The listing builds one solid part. Answer for the finished solid, in the listing's coordinates (mm). A direction names the side the tool comes from. Give positions to 0.01 mm unless a question says otherwise; leave off trailing zeros. Order: outer loops, then holes, each group sorted by start corner. A loop starts at its lowest first (then second) coordinate and runs counter-clockwise, first axis right, second up. Notation, with made-up numbers: (-33.75, 42.5) - (6.25, 42.5) arc R36 cw to (6.25, 77.5) - close; hole circle Ø5 at (6.25, 65.25). An arc over 180 degrees is marked (long way). Write each question's results on one line, items separated by ' | '. Start each with the question number.
1. Determine the mould class of faces 3 (the face through (38, 0, 31)), 4 (the face through (76.2, 2, 14)), 5 (the face through (25.48, 1.61, 50.55)), 6 (the face through (22, 1.6, 21.8)) for opening direction X: released by +X, released by -X, zero draft, split by the parting line, or undercut.
2. Section D-D (y = 1.7) is taken. State how many separate pieces and enclosed holes the cut face has, and give its area (3 significant figures).
3. Flat-ended cylindrical pins translate along their axes: pin 1 (1.5 mm diameter, centred on y = 2.5, z = 26, fed in from +X); pin 2 (3.5 mm diameter, centred on x = 38.1, z = 38.1, fed in from -Y); pin 3 (1 mm diameter, centred on x = 35, y = 1, fed in from -Z); pin 4 (1 mm diameter, centred on y = 1, z = 35, fed in from -X). Find the tip coordinate at first contact, or state that the pin passes through.
4. Section C-C (x = 38.1) is taken. Give the vertices of the cut face in (y, z) (3 decimals).
5. Find the intervals of material crossed by L1, parallel to X at y = 2.1, z = 17.5; L2, parallel to X at y = 2.05, z = 38.1; L3, parallel to Z at x = 46.5, y = 0.75, in increasing order.
6. Section B-B (z = 38.1) is taken. Give the vertices of the cut face in (x, y) (3 decimals).
7. Which of the six approach directions +Z, -Z, +X, -X, +Y, -Y give full straight-line access (tool end or side, diameter ignored) to faces 1 (the face through (63.3, 1.6, 38.3)), 2 (the face through (22.098, 2, 12))?
8. Section A-A (x = 12.7) is taken. Give the vertices of the cut face in (y, z) (3 decimals), and give its area (3 significant figures).
Autodesk Fusion 360 part; units mm, degrees
sketch "Sketch1" plane through (0, 0, 0) normal (0, 1, 0) x (1, 0, 0)
  line L0 (0, 0) -> (0, -25.4)
  line L1 (76.2, -25.4) -> (76.2, 0)
  line L2 (76.2, 0) -> (54.102, 0)
  line L3 (54.102, 0) -> (54.102, -25.4)
  line L4 (54.102, -25.4) -> (22.098, -25.4)
  line L5 (22.098, -25.4) -> (22.098, 0)
  line L6 (22.098, 0) -> (0, 0)
  line L7 (38.1, -25.4) -> (38.1, -50.8) construction
  circle A0 centre (23.7818, -23.7162) radius 2.3813
  line L8 (23.7818, -23.7162) -> (23.7818, -25.4) construction
  line L9 (23.7818, -23.7162) -> (22.098, -23.7162) construction
  circle A1 centre (12.7, -12.7) radius 2.7781
  line L10 (0, -25.4) -> (25.4, -50.8)
  line L11 (25.4, -50.8) -> (50.8, -50.8)
  line L12 (50.8, -50.8) -> (76.2, -25.4)
  circle A2 centre (12.7, -25.4) radius 2.7781
  circle A3 centre (25.4, -38.1) radius 2.7781
  circle A4 centre (38.1, -38.1) radius 2.7781
  circle A5 centre (50.8, -38.1) radius 2.7781
  circle A6 centre (63.5, -12.7) radius 2.7781
  circle A7 centre (63.5, -25.4) radius 2.7781
  circle A8 centre (52.4182, -23.7162) radius 2.3813
  dimension "d1" = 76.2
  dimension "d3" = 32.004
  dimension "d4" = 25.4
  dimension "d6" = 25.4
  dimension "d8" = 4.7625
  dimension "d9" = 5.5563
  dimension "d10" = 12.7
  dimension "d26" = 25.4
  dimension "d43" = 25.4
  dimension "d44" = 12.7
  dimension "d47" = -25.4
  dimension "d48" = -50.8
extrude "Extrude1" add sketch "Sketch1" along normal blind 3.175 contours L0 L1 L2 L3 L4 L5 L6 A0 L10 L11 L12 A8
fillet "Fillet1" radius 3.175 8 edges at (0, 1.5875, 0) (22.098, 1.5875, 0) (54.102, 1.5875, 0) (76.2, 1.5875, 0) (0, 1.5875, 25.4) (25.4, 1.5875, 50.8) (50.8, 1.5875, 50.8) (76.2, 1.5875, 25.4)
fillet "Fillet1" radius 3.175 4 edges at (25.4656, 1.5875, 25.4) (22.098, 1.5875, 22.0324) (50.7344, 1.5875, 25.4) (54.102, 1.5875, 22.0324)
sketch "DXF" plane through (0, 0, 0) normal (0, -1, 0) x (1, 0, 0)
  circle A0 centre (38.1, 38.1) radius 2.7781
  circle A1 centre (12.7, 12.7) radius 2.7781
  circle A2 centre (25.4, 38.1) radius 2.7781
  circle A3 centre (12.7, 25.4) radius 2.7781
  circle A4 centre (63.5, 12.7) radius 2.7781
  circle A5 centre (63.5, 25.4) radius 2.7781
  circle A6 centre (50.8, 38.1) radius 2.7781
  arc A7 (54.5005, 22.5611) -> (54.102, 21.021) centre (57.277, 21.021) ccw
  line L0 (54.102, 21.021) -> (54.102, 3.175)
  arc A8 (54.102, 3.175) -> (57.277, 0) centre (57.277, 3.175) ccw
  line L1 (57.277, 0) -> (73.025, 0)
  arc A9 (73.025, 0) -> (76.2, 3.175) centre (73.025, 3.175) ccw
  line L2 (76.2, 3.175) -> (76.2, 24.0849)
  arc A10 (76.2, 24.0849) -> (75.2701, 26.3299) centre (73.025, 24.0849) ccw
  line L3 (75.2701, 26.3299) -> (51.7299, 49.8701)
  arc A11 (51.7299, 49.8701) -> (49.4849, 50.8) centre (49.4849, 47.625) ccw
  line L4 (49.4849, 50.8) -> (26.7151, 50.8)
  arc A12 (26.7151, 50.8) -> (24.4701, 49.8701) centre (26.7151, 47.625) ccw
  line L5 (24.4701, 49.8701) -> (0.9299, 26.3299)
  arc A13 (0.9299, 26.3299) -> (0, 24.0849) centre (3.175, 24.0849) ccw
  line L6 (0, 24.0849) -> (0, 3.175)
  arc A14 (0, 3.175) -> (3.175, 0) centre (3.175, 3.175) ccw
  line L7 (3.175, 0) -> (18.923, 0)
  arc A15 (18.923, 0) -> (22.098, 3.175) centre (18.923, 3.175) ccw
  line L8 (22.098, 3.175) -> (22.098, 21.021)
  arc A16 (22.098, 21.021) -> (21.6995, 22.5611) centre (18.923, 21.021) ccw
  arc A17 (24.9369, 25.7985) -> (21.6995, 22.5611) centre (23.7818, 23.7162) ccw
  arc A18 (24.9369, 25.7985) -> (26.477, 25.4) centre (26.477, 28.575) ccw
  line L9 (26.477, 25.4) -> (49.723, 25.4)
  arc A19 (49.723, 25.4) -> (51.2631, 25.7985) centre (49.723, 28.575) ccw
  arc A20 (54.5005, 22.5611) -> (51.2631, 25.7985) centre (52.4182, 23.7162) ccw
equation "TOLERANCE = 0.01 in"
equation "d3 = 1 in + 2 * PLATE_THICKNESS + TOLERANCE"
equation "d9 = ( 7 / 32 ) * 1 in"
equation "HOLE_DIAMETER = ( 7 / 32 ) * 1 in"
equation "PLATE_THICKNESS = 0.125 in"
Reported:
1) face 3: zero draft | face 4: released by +X | face 5: released by -X | face 6: undercut
2) separate pieces: 1 | enclosed holes: 7 | area: 2,230 mm²
3) pin 1: x = 75.98 | pin 2: through | pin 3: z = 25.4 | pin 4: x = 9.1
4) outline: (0, 25.4) - (3.175, 25.4) - (3.175, 35.322) - (0, 35.322) - close; (0, 40.878) - (3.175, 40.878) - (3.175, 50.8) - (0, 50.8) - close
5) L1: 0 to 22.1, 54.1 to 76.2 | L2: 12.7 to 22.62, 28.18 to 35.32, 40.88 to 48.02, 53.58 to 63.5 | L3: 25.4 to 50.8
6) outline: (12.7, 0) - (22.622, 0) - (22.622, 3.175) - (12.7, 3.175) - close; (28.178, 0) - (35.322, 0) - (35.322, 3.175) - (28.178, 3.175) - close; (40.878, 0) - (48.022, 0) - (48.022, 3.175) - (40.878, 3.175) - close; (53.578, 0) - (63.5, 0) - (63.5, 3.175) - (53.578, 3.175) - close
7) face 1: +Z, +X, +Y, -Y | face 2: -Z, +Y, -Y
8) outline: (0, 0) - (3.175, 0) - (3.175, 9.922) - (0, 9.922) - close; (0, 15.478) - (3.175, 15.478) - (3.175, 22.622) - (0, 22.622) - close; (0, 28.178) - (3.175, 28.178) - (3.175, 38.1) - (0, 38.1) - close | area: 85.7 mm²
